from build123d import *

# Parameters (mm, degrees)
SKETCH1_R           = 2.6035
BOSS_EXTRUDE1_DEPTH = 63.5


with BuildPart() as part:
    # Sketch1 → Boss-Extrude1 (new body, symmetric)
    with BuildSketch(Plane(origin=(0, 0, 0), x_dir=(0, 0, -1), z_dir=(1, 0, 0))):
        with BuildLine():
            Line((6.333126718, -12.7), (9.550443118, -12.7))
            ThreePointArc((9.550443118, -12.7), (10.058366869, -12.192000006), (10.566443095, -12.699847501))
            ThreePointArc((10.566443095, -12.699847501), (12.082537762, -12.08250727), (12.699846982, -10.566399977))
            ThreePointArc((12.699846982, -10.566399977), (12.192000006, -10.058323491), (12.7, -9.5504))
            Line((12.7, -9.5504), (12.7, -6.3330836))
            ThreePointArc((12.7, -6.3330836), (12.192, -5.8250836), (12.7, -5.3170836))
            Line((12.7, -5.3170836), (12.7, -4.287469289))
            ThreePointArc((12.7, -4.287469289), (12.39275138, -3.545705502), (11.650987593, -3.238456882))
            Line((11.650987593, -3.238456882), (11.539212407, -3.238456882))
            ThreePointArc((11.539212407, -3.238456882), (10.79744862, -3.545705502), (10.4902, -4.287469289))
            Line((10.4902, -4.287469289), (10.4902, -6.402089023))
            ThreePointArc((10.4902, -6.402089023), (9.856505071, -7.351067942), (8.737131347, -7.129408934))
            Line((8.737131347, -7.129408934), (5.441005833, -3.840816462))
            ThreePointArc((5.441005833, -3.840816462), (4.750877967, -2.809883091), (4.5085, -1.593185507))
            Line((4.5085, -1.593185507), (4.5085, 1.593185507))
            ThreePointArc((4.5085, 1.593185507), (4.750877967, 2.809883091), (5.441005833, 3.840816462))
            Line((5.441005833, 3.840816462), (8.737131347, 7.129408934))
            ThreePointArc((8.737131347, 7.129408934), (9.856505071, 7.351067942), (10.4902, 6.402089023))
            Line((10.4902, 6.402089023), (10.4902, 4.287469289))
            ThreePointArc((10.4902, 4.287469289), (10.79744862, 3.545705502), (11.539212407, 3.238456882))
            Line((11.539212407, 3.238456882), (11.650987593, 3.238456882))
            ThreePointArc((11.650987593, 3.238456882), (12.39275138, 3.545705502), (12.7, 4.287469289))
            Line((12.7, 4.287469289), (12.7, 5.3170836))
            ThreePointArc((12.7, 5.3170836), (12.192, 5.8250836), (12.7, 6.3330836))
            Line((12.7, 6.3330836), (12.7, 9.5504))
            ThreePointArc((12.7, 9.5504), (12.192000006, 10.058323491), (12.699846982, 10.566399977))
            ThreePointArc((12.699846982, 10.566399977), (12.082537762, 12.08250727), (10.566443095, 12.699847501))
            ThreePointArc((10.566443095, 12.699847501), (10.058366869, 12.192000006), (9.550443118, 12.7))
            Line((9.550443118, 12.7), (6.333126718, 12.7))
            ThreePointArc((6.333126718, 12.7), (5.825126718, 12.192), (5.317126718, 12.7))
            Line((5.317126718, 12.7), (4.287512407, 12.7))
            ThreePointArc((4.287512407, 12.7), (3.54574862, 12.39275138), (3.2385, 11.650987593))
            Line((3.2385, 11.650987593), (3.2385, 11.539212407))
            ThreePointArc((3.2385, 11.539212407), (3.54574862, 10.79744862), (4.287512407, 10.4902))
            Line((4.287512407, 10.4902), (6.476788598, 10.4902))
            ThreePointArc((6.476788598, 10.4902), (7.432222385, 9.85140422), (7.207036008, 8.724370562))
            Line((7.207036008, 8.724370562), (3.898272566, 5.423169045))
            ThreePointArc((3.898272566, 5.423169045), (2.869120213, 4.736787962), (1.655778399, 4.4958))
            Line((1.655778399, 4.4958), (-1.655778399, 4.4958))
            ThreePointArc((-1.655778399, 4.4958), (-2.869120213, 4.736787962), (-3.898272566, 5.423169045))
            Line((-3.898272566, 5.423169045), (-7.207036008, 8.724370562))
            ThreePointArc((-7.207036008, 8.724370562), (-7.432222385, 9.85140422), (-6.476788598, 10.4902))
            Line((-6.476788598, 10.4902), (-4.287512407, 10.4902))
            ThreePointArc((-4.287512407, 10.4902), (-3.54574862, 10.79744862), (-3.2385, 11.539212407))
            Line((-3.2385, 11.539212407), (-3.2385, 11.650987593))
            ThreePointArc((-3.2385, 11.650987593), (-3.54574862, 12.39275138), (-4.287512407, 12.7))
            Line((-4.287512407, 12.7), (-5.317126718, 12.7))
            ThreePointArc((-5.317126718, 12.7), (-5.825126718, 12.192), (-6.333126718, 12.7))
            Line((-6.333126718, 12.7), (-9.550443118, 12.7))
            ThreePointArc((-9.550443118, 12.7), (-10.058366869, 12.192000006), (-10.566443095, 12.699847501))
            ThreePointArc((-10.566443095, 12.699847501), (-12.082537762, 12.08250727), (-12.699846982, 10.566399977))
            ThreePointArc((-12.699846982, 10.566399977), (-12.192000006, 10.058323491), (-12.7, 9.5504))
            Line((-12.7, 9.5504), (-12.7, 6.3330836))
            ThreePointArc((-12.7, 6.3330836), (-12.192, 5.8250836), (-12.7, 5.3170836))
            Line((-12.7, 5.3170836), (-12.7, 4.287469289))
            ThreePointArc((-12.7, 4.287469289), (-12.39275138, 3.545705502), (-11.650987593, 3.238456882))
            Line((-11.650987593, 3.238456882), (-11.539212407, 3.238456882))
            ThreePointArc((-11.539212407, 3.238456882), (-10.79744862, 3.545705502), (-10.4902, 4.287469289))
            Line((-10.4902, 4.287469289), (-10.4902, 6.402089023))
            ThreePointArc((-10.4902, 6.402089023), (-9.856505071, 7.351067942), (-8.737131347, 7.129408934))
            Line((-8.737131347, 7.129408934), (-5.441005833, 3.840816462))
            ThreePointArc((-5.441005833, 3.840816462), (-4.750877967, 2.809883091), (-4.5085, 1.593185507))
            Line((-4.5085, 1.593185507), (-4.5085, -1.593185507))
            ThreePointArc((-4.5085, -1.593185507), (-4.750877967, -2.809883091), (-5.441005833, -3.840816462))
            Line((-5.441005833, -3.840816462), (-8.737131347, -7.129408934))
            ThreePointArc((-8.737131347, -7.129408934), (-9.856505071, -7.351067942), (-10.4902, -6.402089023))
            Line((-10.4902, -6.402089023), (-10.4902, -4.287469289))
            ThreePointArc((-10.4902, -4.287469289), (-10.79744862, -3.545705502), (-11.539212407, -3.238456882))
            Line((-11.539212407, -3.238456882), (-11.650987593, -3.238456882))
            ThreePointArc((-11.650987593, -3.238456882), (-12.39275138, -3.545705502), (-12.7, -4.287469289))
            Line((-12.7, -4.287469289), (-12.7, -5.3170836))
            ThreePointArc((-12.7, -5.3170836), (-12.192, -5.8250836), (-12.7, -6.3330836))
            Line((-12.7, -6.3330836), (-12.7, -9.5504))
            ThreePointArc((-12.7, -9.5504), (-12.192000006, -10.058323491), (-12.699846982, -10.566399977))
            ThreePointArc((-12.699846982, -10.566399977), (-12.082537762, -12.08250727), (-10.566443095, -12.699847501))
            ThreePointArc((-10.566443095, -12.699847501), (-10.058366869, -12.192000006), (-9.550443118, -12.7))
            Line((-9.550443118, -12.7), (-6.333126718, -12.7))
            ThreePointArc((-6.333126718, -12.7), (-5.825126718, -12.192), (-5.317126718, -12.7))
            Line((-5.317126718, -12.7), (-4.287512407, -12.7))
            ThreePointArc((-4.287512407, -12.7), (-3.54574862, -12.39275138), (-3.2385, -11.650987593))
            Line((-3.2385, -11.650987593), (-3.2385, -11.539212407))
            ThreePointArc((-3.2385, -11.539212407), (-3.54574862, -10.79744862), (-4.287512407, -10.4902))
            Line((-4.287512407, -10.4902), (-6.416408329, -10.4902))
            ThreePointArc((-6.416408329, -10.4902), (-7.41473083, -9.822813117), (-7.179650497, -8.645192506))
            Line((-7.179650497, -8.645192506), (-3.952270251, -5.423690499))
            ThreePointArc((-3.952270251, -5.423690499), (-2.922936451, -4.736929036), (-1.709253557, -4.4958))
            Line((-1.709253557, -4.4958), (1.709253557, -4.4958))
            ThreePointArc((1.709253557, -4.4958), (2.922936451, -4.736929036), (3.952270251, -5.423690499))
            Line((3.952270251, -5.423690499), (7.179650497, -8.645192506))
            ThreePointArc((7.179650497, -8.645192506), (7.41473083, -9.822813117), (6.416408329, -10.4902))
            Line((6.416408329, -10.4902), (4.287512407, -10.4902))
            ThreePointArc((4.287512407, -10.4902), (3.54574862, -10.79744862), (3.2385, -11.539212407))
            Line((3.2385, -11.539212407), (3.2385, -11.650987593))
            ThreePointArc((3.2385, -11.650987593), (3.54574862, -12.39275138), (4.287512407, -12.7))
            Line((4.287512407, -12.7), (5.317126718, -12.7))
            ThreePointArc((5.317126718, -12.7), (5.825126718, -12.192), (6.333126718, -12.7))
        make_face()
        Circle(SKETCH1_R, mode=Mode.SUBTRACT)
    extrude(amount=BOSS_EXTRUDE1_DEPTH, both=True)


solid = part.part
The model under review builds one solid part; all positions refer to its coordinate system, in mm. A direction names the side the tool comes from. Give positions to 0.01 mm unless a question says otherwise; leave off trailing zeros. Order: outer loops, then holes, each group sorted by start corner. A loop starts at its lowest first (then second) coordinate and runs counter-clockwise, first axis right, second up. Notation, with made-up numbers: M 82,59.5 L 86,59.5 A26 ccw 86,81.5 Z; hole C 9.5,72 d5. An arc over 180 degrees is marked long. Answer in a Markdown table with one row per item. Add a question column.
1. Machinability: for faces 1 (the flat face through (1, 5, 10.49)), 2 (the flat face through (1, -8, -12.7)), 3 (the flat face through (1, -4.496, 0)), which of the approach directions +Z, -Z, +X, -X, +Y, -Y give a long, thin tool a straight path to every point of the face, cutting with its end or side? Answer none if there is none.
2. For pin 1 Ø2 at (y, z) = (-10, 6.5) entering from +X; pin 2 Ø4 at (x, z) = (10.5, -0.5) entering from +Y; pin 3 Ø2.5 at (x, z) = (-18, 0) entering from -Y; pin 4 Ø2.5 at (x, z) = (-5.5, 0.5) entering from +Y, all flat-tipped, find the tip position at first contact; note any pin that passes through.
3. Add section A-A on z = 0. State the section outline as (x, y) points, plus the area to 3 significant figures.
4. Mouldability with a two-part tool opening along Z and no side actions: class faces 4 (the flat face through (-63.5, 3, 0)), 5 (the flat face through (1, 0, -4.508)), 6 (the flat face through (0.889, 5.462, -7.066)) as released by +Z, released by -Z, zero draft, split by the parting line, or undercut.
5. To check wall thickness, follow line 1 along Y through (x, z) = (-6, -4.25); line 2 along Y through (x, z) = (5, 0); line 3 along Y through (x, z) = (13, -6.5). State the ranges of each line that lie inside material, in increasing order.
6. Add section B-B on y = 0. State the section outline as (x, z) points, plus the area to 3 significant figures.
The answers:
| question | item | result |
|---|---|---|
| 1 | face 1 | +X, -X |
| 1 | face 2 | -Z, +X, -X, +Y, -Y |
| 1 | face 3 | +X, -X, -Y |
| 2 | pin 1 | x = 63.5 |
| 2 | pin 2 | y = 4.61 |
| 2 | pin 3 | y = -4.5 |
| 2 | pin 4 | y = 4.5 |
| 3 | outline | M -63.5,-4.5 L 63.5,-4.5 L 63.5,-2.6 L -63.5,-2.6 Z; M -63.5,2.6 L 63.5,2.6 L 63.5,4.5 L -63.5,4.5 Z |
| 3 | area | 481 mm2 |
| 4 | face 4 | zero draft |
| 4 | face 5 | released by -Z |
| 4 | face 6 | undercut |
| 5 | line 1 | -12.7 to -10.49, -5.72 to 5.77, 10.49 to 12.7 |
| 5 | line 2 | -4.5 to -2.6, 2.6 to 4.5 |
| 5 | line 3 | -12.7 to -10.49, -7.97 to -4.9, 4.9 to 8.02, 10.49 to 12.7 |
| 6 | outline | M -63.5,-4.51 L 63.5,-4.51 L 63.5,-2.6 L -63.5,-2.6 Z; M -63.5,2.6 L 63.5,2.6 L 63.5,4.51 L -63.5,4.51 Z |
| 6 | area | 484 mm2 |
